Can you work these out from the model? Positions are in its coordinate system, mm. A direction names the side the tool comes from. Give positions to 0.01 mm unless a question says otherwise; leave off trailing zeros. Order: outer loops, then holes, each group sorted by start corner. A loop starts at its lowest first (then second) coordinate and runs counter-clockwise, first axis right, second up. Notation, with made-up numbers: (9.25, 88.5) - (64.25, 88.5) arc R5 cw to (64.25, 92.5) - close; hole circle Ø2 at (67, -26). An arc over 180 degrees is marked (long way). Answer as a JSON object with one key per item and string values.
```python
from build123d import *

# Parameters (mm, degrees)
SKETCH1_W           = 76
SKETCH1_H           = 54.8
BOSS_EXTRUDE1_DEPTH = 3.2
CUT_EXTRUDE1_START  = 1.2
SKETCH2_W           = 1.2
SKETCH2_H           = 1.2
CUT_EXTRUDE1_DEPTH  = 73.6
CUT_EXTRUDE2_START  = 76
SKETCH3_R           = 0.8
CUT_EXTRUDE2_DEPTH  = 10


with BuildPart() as part:
    # Sketch1 → Boss-Extrude1 (new body)
    with BuildSketch(Plane.XY):
        with Locations((38, -27.4)):
            Rectangle(SKETCH1_W, SKETCH1_H)
    extrude(amount=BOSS_EXTRUDE1_DEPTH)

    # Sketch2 → Cut-Extrude1 (cut)
    with BuildSketch(Plane(origin=(0, 0, 0), x_dir=(0, 0, -1), z_dir=(1, 0, 0)).offset(CUT_EXTRUDE1_START)):
        with Locations((-2.6, -13.6)):
            Rectangle(SKETCH2_W, SKETCH2_H)
        with Locations((-2.6, -26.8)):
            Rectangle(SKETCH2_W, SKETCH2_H)
        with Locations((-2.6, -40)):
            Rectangle(SKETCH2_W, SKETCH2_H)
        with Locations((-2.6, -53.2)):
            Rectangle(SKETCH2_W, SKETCH2_H)
    extrude(amount=CUT_EXTRUDE1_DEPTH, mode=Mode.SUBTRACT)

    # Sketch3 → Cut-Extrude2 (cut)
    with BuildSketch(Plane(origin=(0, 0, 0), x_dir=(0, 0, -1), z_dir=(1, 0, 0)).offset(CUT_EXTRUDE2_START)):
        with Locations((-1.6, -7)):
            Circle(SKETCH3_R)
        with Locations((-1.6, -20.2)):
            Circle(SKETCH3_R)
        with Locations((-1.6, -33.998867877)):
            Circle(SKETCH3_R)
        with Locations((-1.6, -46.6)):
            Circle(SKETCH3_R)
    extrude(amount=-CUT_EXTRUDE2_DEPTH, mode=Mode.SUBTRACT)


solid = part.part
```
Q1. If we section it at B-B, the plane x = 9.5: Please give me the cut outline in (y, z), then the cut area to 3 significant figures.
Recorded:
{"outline": "(-54.8, 0) - (0, 0) - (0, 3.2) - (-13, 3.2) - (-13, 2) - (-14.2, 2) - (-14.2, 3.2) - (-26.2, 3.2) - (-26.2, 2) - (-27.4, 2) - (-27.4, 3.2) - (-39.4, 3.2) - (-39.4, 2) - (-40.6, 2) - (-40.6, 3.2) - (-52.6, 3.2) - (-52.6, 2) - (-53.8, 2) - (-53.8, 3.2) - (-54.8, 3.2) - close", "area": "170 mm^2"}
Q2. I need wall thicknesses on L1, parallel to Y at x = 71.5, z = 1.6; L2, parallel to Y at x = 40, z = 2.35; L3, parallel to Z at x = 68.75, y = -46.6. Which ranges of each line are inside material? Lowest first, please.
Recorded:
{"L1": "y = -54.8 to -47.4, -45.8 to -34.8, -33.2 to -21, -19.4 to -7.8, -6.2 to 0", "L2": "y = -54.8 to -53.8, -52.6 to -40.6, -39.4 to -27.4, -26.2 to -14.2, -13 to 0", "L3": "z = 0 to 0.8, 2.4 to 3.2"}
Q3. If we section it at A-A, the plane y = -7: Please give me the cut outline in (x, z).
Recorded:
{"outline": "(0, 0) - (76, 0) - (76, 0.8) - (66, 0.8) - (66, 2.4) - (76, 2.4) - (76, 3.2) - (0, 3.2) - close"}
Q4. If we section it at C-C, the plane x = 69.5: Please give me the cut outline in (y, z).
Recorded:
{"outline": "(-54.8, 0) - (0, 0) - (0, 3.2) - (-13, 3.2) - (-13, 2) - (-14.2, 2) - (-14.2, 3.2) - (-26.2, 3.2) - (-26.2, 2) - (-27.4, 2) - (-27.4, 3.2) - (-39.4, 3.2) - (-39.4, 2) - (-40.6, 2) - (-40.6, 3.2) - (-52.6, 3.2) - (-52.6, 2) - (-53.8, 2) - (-53.8, 3.2) - (-54.8, 3.2) - close; hole circle Ø1.6 at (-46.6, 1.6); hole circle Ø1.6 at (-34, 1.6); hole circle Ø1.6 at (-20.2, 1.6); hole circle Ø1.6 at (-7, 1.6)"}
Q5. Which directions (+Z, -Z, +X, -X, +Y, -Y) give clear straight access to the entire face, cutting with the end or side of a thin tool? Please do faces 1 (the face through (66, -47, 2)), 2 (the face through (37, -54.8, 2)).
Recorded:
{"face 1": "+X", "face 2": "+Z, -Z, +X, -X, -Y"}
Q6. I'm going to push flat-ended pins straight in: pin 1 Ø0.5 at (y, z) = (-46.5, 1.5) entering from +X; pin 2 Ø8 at (x, y) = (15, -23.5) entering from -Z; pin 3 Ø1 at (x, y) = (24.5, -40) entering from +Z. Where does each tip first touch, or does it pass through?
Recorded:
{"pin 1": "stops at x = 66", "pin 2": "stops at z = 0", "pin 3": "stops at z = 2"}
